from build123d import *

# Parameters (mm, degrees)
SKETCH1_R           = 24.16125
SKETCH1_R_2         = 28.9935
BOSS_EXTRUDE1_DEPTH = 5
SCALE1_SCALE        = 1.5
SKETCH2_R           = 5
CUT_EXTRUDE1_DEPTH  = 10


with BuildPart() as part:
    # Sketch1 → Boss-Extrude1 (new body)
    with BuildSketch(Plane(origin=(0, 0, 0), x_dir=(0, 0, -1), z_dir=(1, 0, 0))):
        with BuildLine():
            Line((116, 50.1), (116, -50.1))
            ThreePointArc((116, -50.1), (0, -166.1), (-116, -50.1))
            Line((-116, -50.1), (-116, 50.1))
            ThreePointArc((-116, 50.1), (0, 166.1), (116, 50.1))
        make_face()
        with Locations((0, 61.077179293)):
            Circle(SKETCH1_R, mode=Mode.SUBTRACT)
        with Locations((0, -51.244320707)):
            Circle(SKETCH1_R_2, mode=Mode.SUBTRACT)
    extrude(amount=BOSS_EXTRUDE1_DEPTH)


with BuildPart() as part_1:
    # Scale1: scaled about (2.5, 0.381982972, 0)
    add(part.part.scale(SCALE1_SCALE).moved(Location((-1.25, -0.190991486, 0))))

    # Sketch2 → Cut-Extrude1 (cut)
    with BuildSketch(Plane(origin=(6.25, 0, 0), x_dir=(0, 0, -1), z_dir=(1, 0, 0))):
        with Locations((116.5, -58.057472547)):
            Circle(SKETCH2_R)
        with Locations((116.5, -77.057472547)):
            Circle(SKETCH2_R)
        with Locations((114.516366113, -98.464291372)):
            Circle(SKETCH2_R)
        with Locations((108.633014726, -119.142126657)):
            Circle(SKETCH2_R)
        with Locations((116.5, -20.057472547)):
            Circle(SKETCH2_R)
        with Locations((116.5, -1.057472547)):
            Circle(SKETCH2_R)
        with Locations((116.5, 17.942527453)):
            Circle(SKETCH2_R)
        with Locations((116.5, 36.942527453)):
            Circle(SKETCH2_R)
        with Locations((116.5, 55.942527453)):
            Circle(SKETCH2_R)
        with Locations((116.5, 74.942527453)):
            Circle(SKETCH2_R)
        with Locations((116.5, 91.424777453)):
            Circle(SKETCH2_R)
        with Locations((114.516366113, 112.831596279)):
            Circle(SKETCH2_R)
        with Locations((108.633014726, 133.509431564)):
            Circle(SKETCH2_R)
        with Locations((86.094538856, 169.910319938)):
            Circle(SKETCH2_R)
        with Locations((70.206935138, 184.393784431)):
            Circle(SKETCH2_R)
        with Locations((51.928518448, 195.711300896)):
            Circle(SKETCH2_R)
        with Locations((31.881738343, 203.477464883)):
            Circle(SKETCH2_R)
        with Locations((10.749263877, 207.427808992)):
            Circle(SKETCH2_R)
        with Locations((-10.749263877, 207.427808992)):
            Circle(SKETCH2_R)
        with Locations((-31.881738343, 203.477464883)):
            Circle(SKETCH2_R)
        with Locations((-51.928518448, 195.711300896)):
            Circle(SKETCH2_R)
        with Locations((-70.206935138, 184.393784431)):
            Circle(SKETCH2_R)
        with Locations((-86.094538856, 169.910319938)):
            Circle(SKETCH2_R)
        with Locations((-99.050296312, 152.754124429)):
            Circle(SKETCH2_R)
        with Locations((-108.633014726, 133.509431564)):
            Circle(SKETCH2_R)
        with Locations((-114.516366113, 112.831596279)):
            Circle(SKETCH2_R)
        with Locations((-116.5, 91.424777453)):
            Circle(SKETCH2_R)
        with Locations((-116.5, 74.942527453)):
            Circle(SKETCH2_R)
        with Locations((-116.5, 55.942527453)):
            Circle(SKETCH2_R)
        with Locations((-116.5, 36.942527453)):
            Circle(SKETCH2_R)
        with Locations((-116.5, 17.942527453)):
            Circle(SKETCH2_R)
        with Locations((-116.5, -1.057472547)):
            Circle(SKETCH2_R)
        with Locations((-116.5, -20.057472547)):
            Circle(SKETCH2_R)
        with Locations((-116.5, -39.057472547)):
            Circle(SKETCH2_R)
        with Locations((-116.5, -58.057472547)):
            Circle(SKETCH2_R)
        with Locations((-116.5, -77.057472547)):
            Circle(SKETCH2_R)
        with Locations((-114.516366113, -98.464291372)):
            Circle(SKETCH2_R)
        with Locations((-108.633014726, -119.142126657)):
            Circle(SKETCH2_R)
        with Locations((-99.050296312, -138.386819522)):
            Circle(SKETCH2_R)
        with Locations((-86.094538856, -155.543015032)):
            Circle(SKETCH2_R)
        with Locations((-70.206935138, -170.026479525)):
            Circle(SKETCH2_R)
        with Locations((-51.928518448, -181.34399599)):
            Circle(SKETCH2_R)
        with Locations((-31.881738343, -189.110159976)):
            Circle(SKETCH2_R)
        with Locations((-10.749263877, -193.060504085)):
            Circle(SKETCH2_R)
        with Locations((10.749263877, -193.060504085)):
            Circle(SKETCH2_R)
        with Locations((31.881738343, -189.110159976)):
            Circle(SKETCH2_R)
        with Locations((51.928518448, -181.34399599)):
            Circle(SKETCH2_R)
        with Locations((70.206935138, -170.026479525)):
            Circle(SKETCH2_R)
        with Locations((99.050296313, -138.386819522)):
            Circle(SKETCH2_R)
        with Locations((86.094538856, -155.543015031)):
            Circle(SKETCH2_R)
        with Locations((116.5, -39.057472547)):
            Circle(SKETCH2_R)
        with Locations((99.050296313, 152.754124429)):
            Circle(SKETCH2_R)
    extrude(amount=-CUT_EXTRUDE1_DEPTH, mode=Mode.SUBTRACT)


solid = part_1.part
Geometry check sheet. Reference: the model listing, model coordinates, mm. Coordinates: 2 decimals unless noted, no trailing zeros. Order: outer loops, then holes, each group sorted by start corner. A loop starts at its lowest first (then second) coordinate and runs counter-clockwise, first axis right, second up. Notation, with made-up numbers: (49.5, 28.25) - (99.5, 28.25) arc R22 ccw to (99.5, 57.25) - close; hole circle Ø5 at (11.5, 33). An arc over 180 degrees is marked (long way). One line per item, written item: value.
(1) Thickness scan on probe 1 along Y at (x, z) = (0.5, -89.5); probe 2 along Z at (x, y) = (4, -187); probe 3 along Z at (x, y) = (3.25, 169.5). Record the ranges inside material, lowest first. Write a range as from..to.
Data:
probe 1: y = -224.56..-159.2, -151.88..166.25, 173.57..224.18
probe 2: z = -133.45..-36.41, -27.35..27.35, 36.41..133.45
probe 3: z = -146.08..-91.08, -81.11..81.11, 91.08..146.08
(2) Release check for a two-part mould opening along Z. For faces 1 (the face through (2.448, 248.917, 3.826)), 2 (the face through (2.552, 135.011, 103.864)), 3 (the face through (-1.25, 3, -2)) record: +Z half, -Z half, draft (parallel to the pull), parting line (faces both ways), or undercut.
Data:
face 1: parting line
face 2: undercut
face 3: draft
(3) Sectioned sample at A-A (z = -147). Enter the section's corners in (x, y), and give its area (3 significant figures).
Data:
outline: (-1.25, -168.44) - (6.25, -168.44) - (6.25, 168.06) - (-1.25, 168.06) - close
area: 2,520 mm^2
(4) Depth check by flat-ended pin: pin 1 Ø3 at (x, z) = (5, -60) entering from -Y; pin 2 Ø1.5 at (x, z) = (1, 46) entering from -Y; pin 3 Ø1 at (x, y) = (-0.5, -141.5) entering from +Z. Enter the tip coordinate at first touch or a pass-through.
Data:
pin 1: stops at y = -239.21
pin 2: stops at y = -243.35
pin 3: stops at z = 161.14
(5) Sectioned sample at B-B (x = 4.25). Count the separate pieces of the cut face and the enclosed holes in it, and give its area (3 significant figures).
Data:
separate pieces: 1
enclosed holes: 54
area: 133,000 mm^2
